from build123d import *

# Parameters (mm, degrees)
EXTRUDE_1_DEPTH     = 19.2
SKETCH_9_W          = 230
SKETCH_9_H          = 17.5
SKETCH_9_R          = 2.1
EXTRUDE_2_DEPTH     = 3
SKETCH_13_W         = 230
SKETCH_13_H         = 16
SKETCH_13_R         = 2.1
EXTRUDE_3_DEPTH     = 1.55
SKETCH_14_W         = 230
SKETCH_14_H         = 47.5
SKETCH_14_R         = 2.1
EXTRUDE_4_DEPTH     = 3
SKETCH_15_W         = 208.313471068
SKETCH_15_H         = 9.29970853
EXTRUDE_5_DEPTH     = 47.5
SKETCH_16_W         = 230
SKETCH_16_H         = 33.21324475
EXTRUDE_6_DEPTH     = 3
SKETCH_18_W         = 230
SKETCH_18_H         = 20.5
EXTRUDE_7_DEPTH     = 44.5
SKETCH_19_W         = 230
SKETCH_19_H         = 8.5
CUT_EXTRUDE_1_DEPTH = 236.542459017
CUT_EXTRUDE_2_DEPTH = 20.75


with BuildPart() as part:
    # ｽｹｯﾁ5 → ﾎﾞｽ - 押し出し1 (new body)
    with BuildSketch(Plane.XY.offset(-1.55)):
        with BuildLine():
            Line((230, -2.976), (227.539284327, -2.976))
            ThreePointArc((227.539284327, -2.976), (226.75348461, -2.728238301), (226.251905437, -2.074567596))
            Line((226.251905437, -2.074567596), (225.496824583, 0))
            Line((225.496824583, 0), (219.003175417, 0))
            Line((219.003175417, 0), (218.248094563, -2.074567596))
            ThreePointArc((218.248094563, -2.074567596), (217.74651539, -2.728238301), (216.960715673, -2.976))
            Line((216.960715673, -2.976), (214.839284327, -2.976))
            ThreePointArc((214.839284327, -2.976), (214.05348461, -2.728238301), (213.551905437, -2.074567596))
            Line((213.551905437, -2.074567596), (212.796824583, 0))
            Line((212.796824583, 0), (206.303175417, 0))
            Line((206.303175417, 0), (205.548094563, -2.074567596))
            ThreePointArc((205.548094563, -2.074567596), (205.04651539, -2.728238301), (204.260715673, -2.976))
            Line((204.260715673, -2.976), (202.139284327, -2.976))
            ThreePointArc((202.139284327, -2.976), (201.35348461, -2.728238301), (200.851905437, -2.074567596))
            Line((200.851905437, -2.074567596), (200.096824583, 0))
            Line((200.096824583, 0), (193.603175417, 0))
            Line((193.603175417, 0), (192.848094563, -2.074567596))
            ThreePointArc((192.848094563, -2.074567596), (192.34651539, -2.728238301), (191.560715673, -2.976))
            Line((191.560715673, -2.976), (189.439284327, -2.976))
            ThreePointArc((189.439284327, -2.976), (188.65348461, -2.728238301), (188.151905437, -2.074567596))
            Line((188.151905437, -2.074567596), (187.396824583, 0))
            Line((187.396824583, 0), (180.903175417, 0))
            Line((180.903175417, 0), (180.148094563, -2.074567596))
            ThreePointArc((180.148094563, -2.074567596), (179.64651539, -2.728238301), (178.860715673, -2.976))
            Line((178.860715673, -2.976), (176.739284327, -2.976))
            ThreePointArc((176.739284327, -2.976), (175.95348461, -2.728238301), (175.451905437, -2.074567596))
            Line((175.451905437, -2.074567596), (174.696824583, 0))
            Line((174.696824583, 0), (168.203175417, 0))
            Line((168.203175417, 0), (167.448094563, -2.074567596))
            ThreePointArc((167.448094563, -2.074567596), (166.94651539, -2.728238301), (166.160715673, -2.976))
            Line((166.160715673, -2.976), (164.039284327, -2.976))
            ThreePointArc((164.039284327, -2.976), (163.25348461, -2.728238301), (162.751905437, -2.074567596))
            Line((162.751905437, -2.074567596), (161.996824583, 0))
            Line((161.996824583, 0), (155.503175417, 0))
            Line((155.503175417, 0), (154.748094563, -2.074567596))
            ThreePointArc((154.748094563, -2.074567596), (154.24651539, -2.728238301), (153.460715673, -2.976))
            Line((153.460715673, -2.976), (151.339284327, -2.976))
            ThreePointArc((151.339284327, -2.976), (150.55348461, -2.728238301), (150.051905437, -2.074567596))
            Line((150.051905437, -2.074567596), (149.296824583, 0))
            Line((149.296824583, 0), (142.803175417, 0))
            Line((142.803175417, 0), (142.048094563, -2.074567596))
            ThreePointArc((142.048094563, -2.074567596), (141.54651539, -2.728238301), (140.760715673, -2.976))
            Line((140.760715673, -2.976), (138.639284327, -2.976))
            ThreePointArc((138.639284327, -2.976), (137.85348461, -2.728238301), (137.351905437, -2.074567596))
            Line((137.351905437, -2.074567596), (136.596824583, 0))
            Line((136.596824583, 0), (130.103175417, 0))
            Line((130.103175417, 0), (129.348094563, -2.074567596))
            ThreePointArc((129.348094563, -2.074567596), (128.84651539, -2.728238301), (128.060715673, -2.976))
            Line((128.060715673, -2.976), (125.939284327, -2.976))
            ThreePointArc((125.939284327, -2.976), (125.15348461, -2.728238301), (124.651905437, -2.074567596))
            Line((124.651905437, -2.074567596), (123.896824583, 0))
            Line((123.896824583, 0), (117.403175417, 0))
            Line((117.403175417, 0), (116.648094563, -2.074567596))
            ThreePointArc((116.648094563, -2.074567596), (116.14651539, -2.728238301), (115.360715673, -2.976))
            Line((115.360715673, -2.976), (113.239284327, -2.976))
            ThreePointArc((113.239284327, -2.976), (112.45348461, -2.728238301), (111.951905437, -2.074567596))
            Line((111.951905437, -2.074567596), (111.196824583, 0))
            Line((111.196824583, 0), (104.703175417, 0))
            Line((104.703175417, 0), (103.948094563, -2.074567596))
            ThreePointArc((103.948094563, -2.074567596), (103.44651539, -2.728238301), (102.660715673, -2.976))
            Line((102.660715673, -2.976), (100.539284327, -2.976))
            ThreePointArc((100.539284327, -2.976), (99.75348461, -2.728238301), (99.251905437, -2.074567596))
            Line((99.251905437, -2.074567596), (98.496824583, 0))
            Line((98.496824583, 0), (92.003175417, 0))
            Line((92.003175417, 0), (91.248094563, -2.074567596))
            ThreePointArc((91.248094563, -2.074567596), (90.74651539, -2.728238301), (89.960715673, -2.976))
            Line((89.960715673, -2.976), (87.839284327, -2.976))
            ThreePointArc((87.839284327, -2.976), (87.05348461, -2.728238301), (86.551905437, -2.074567596))
            Line((86.551905437, -2.074567596), (85.796824583, 0))
            Line((85.796824583, 0), (79.303175417, 0))
            Line((79.303175417, 0), (78.548094563, -2.074567596))
            ThreePointArc((78.548094563, -2.074567596), (78.04651539, -2.728238301), (77.260715673, -2.976))
            Line((77.260715673, -2.976), (75.139284327, -2.976))
            ThreePointArc((75.139284327, -2.976), (74.35348461, -2.728238301), (73.851905437, -2.074567596))
            Line((73.851905437, -2.074567596), (73.096824583, 0))
            Line((73.096824583, 0), (66.603175417, 0))
            Line((66.603175417, 0), (65.848094563, -2.074567596))
            ThreePointArc((65.848094563, -2.074567596), (65.34651539, -2.728238301), (64.560715673, -2.976))
            Line((64.560715673, -2.976), (62.439284327, -2.976))
            ThreePointArc((62.439284327, -2.976), (61.65348461, -2.728238301), (61.151905437, -2.074567596))
            Line((61.151905437, -2.074567596), (60.396824583, 0))
            Line((60.396824583, 0), (53.903175417, 0))
            Line((53.903175417, 0), (53.148094563, -2.074567596))
            ThreePointArc((53.148094563, -2.074567596), (52.64651539, -2.728238301), (51.860715673, -2.976))
            Line((51.860715673, -2.976), (49.739284327, -2.976))
            ThreePointArc((49.739284327, -2.976), (48.95348461, -2.728238301), (48.451905437, -2.074567596))
            Line((48.451905437, -2.074567596), (47.696824583, 0))
            Line((47.696824583, 0), (41.203175417, 0))
            Line((41.203175417, 0), (40.448094563, -2.074567596))
            ThreePointArc((40.448094563, -2.074567596), (39.94651539, -2.728238301), (39.160715673, -2.976))
            Line((39.160715673, -2.976), (37.039284327, -2.976))
            ThreePointArc((37.039284327, -2.976), (36.25348461, -2.728238301), (35.751905437, -2.074567596))
            Line((35.751905437, -2.074567596), (34.996824583, 0))
            Line((34.996824583, 0), (28.503175417, 0))
            Line((28.503175417, 0), (27.748094563, -2.074567596))
            ThreePointArc((27.748094563, -2.074567596), (27.24651539, -2.728238301), (26.460715673, -2.976))
            Line((26.460715673, -2.976), (24.339284327, -2.976))
            ThreePointArc((24.339284327, -2.976), (23.55348461, -2.728238301), (23.051905437, -2.074567596))
            Line((23.051905437, -2.074567596), (22.296824583, 0))
            Line((22.296824583, 0), (15.803175417, 0))
            Line((15.803175417, 0), (15.048094563, -2.074567596))
            ThreePointArc((15.048094563, -2.074567596), (14.54651539, -2.728238301), (13.760715673, -2.976))
            Line((13.760715673, -2.976), (11.639284327, -2.976))
            ThreePointArc((11.639284327, -2.976), (10.85348461, -2.728238301), (10.351905437, -2.074567596))
            Line((10.351905437, -2.074567596), (9.596824583, 0))
            Line((9.596824583, 0), (3.103175417, 0))
            Line((3.103175417, 0), (2.348094563, -2.074567596))
            ThreePointArc((2.348094563, -2.074567596), (1.84651539, -2.728238301), (1.060715673, -2.976))
            Line((1.060715673, -2.976), (0, -2.976))
            Line((0, -2.976), (0, -15))
            Line((0, -15), (230, -15))
            Line((230, -15), (230, -2.976))
        make_face()
    extrude(amount=-EXTRUDE_1_DEPTH)


with BuildPart() as body_2:
    # ｽｹｯﾁ9 → ﾎﾞｽ - 押し出し2 (new body)
    with BuildSketch(Plane(origin=(0, 0, -20.75), x_dir=(-1, 0, 0), z_dir=(0, 0, -1))):
        with Locations((-115, -6.25)):
            Rectangle(SKETCH_9_W, SKETCH_9_H)
        with Locations((-25, -7)):
            Circle(SKETCH_9_R, mode=Mode.SUBTRACT)
        with Locations((-85, -7)):
            Circle(SKETCH_9_R, mode=Mode.SUBTRACT)
        with Locations(Location((-145, -7, 0), (0, 0, 180))):
            Circle(SKETCH_9_R, mode=Mode.SUBTRACT)
        with Locations(Location((-205, -7, 0), (0, 0, 180))):
            Circle(SKETCH_9_R, mode=Mode.SUBTRACT)
    extrude(amount=EXTRUDE_2_DEPTH)


with BuildPart() as body_3:
    # ｽｹｯﾁ13 → ﾎﾞｽ - 押し出し3 (new, symmetric)
    with BuildSketch(Plane.XY):
        with Locations((115, -7)):
            Rectangle(SKETCH_13_W, SKETCH_13_H)
        with Locations(Location((85, -7, 0), (0, 0, 180))):
            Circle(SKETCH_13_R, mode=Mode.SUBTRACT)
        with Locations(Location((25, -7, 0), (0, 0, 180))):
            Circle(SKETCH_13_R, mode=Mode.SUBTRACT)
        with Locations((205, -7)):
            Circle(SKETCH_13_R, mode=Mode.SUBTRACT)
        with Locations((145, -7)):
            Circle(SKETCH_13_R, mode=Mode.SUBTRACT)
    extrude(amount=EXTRUDE_3_DEPTH, both=True)


with BuildPart() as body_4:
    # ﾐﾗｰ1: mirrored copy
    add(part.part.mirror(Plane.XY))


with BuildPart() as body_5:
    # Mirror 1 2: mirrored copy
    add(body_2.part.mirror(Plane.XY))


with BuildPart() as body_6:
    # ｽｹｯﾁ14 → ﾎﾞｽ - 押し出し4 (new body)
    with BuildSketch(Plane.XZ.offset(15)):
        with Locations((115, 0)):
            Rectangle(SKETCH_14_W, SKETCH_14_H)
        with Locations(Location((7, 11.15, 0), (0, 0, 180))):
            Circle(SKETCH_14_R, mode=Mode.SUBTRACT)
        with Locations((121.5, -11.15)):
            Circle(SKETCH_14_R, mode=Mode.SUBTRACT)
        with Locations((223, -11.15)):
            Circle(SKETCH_14_R, mode=Mode.SUBTRACT)
        with Locations((7, -11.15)):
            Circle(SKETCH_14_R, mode=Mode.SUBTRACT)
        with Locations(Location((223, 11.15, 0), (0, 0, 180))):
            Circle(SKETCH_14_R, mode=Mode.SUBTRACT)
        with Locations(Location((121.5, 11.15, 0), (0, 0, 180))):
            Circle(SKETCH_14_R, mode=Mode.SUBTRACT)
    extrude(amount=EXTRUDE_4_DEPTH)


with BuildPart() as body_4_1:
    add(body_4.part)

    # Combine 2: union part, body 5, body 6, body 3, body 2
    add(part.part)
    add(body_5.part)
    add(body_6.part)
    add(body_3.part)
    add(body_2.part)

    # ｽｹｯﾁ15 → ﾎﾞｽ - 押し出し5 (add)
    with BuildSketch(Plane(origin=(0, 0, -23.75), x_dir=(-1, 0, 0), z_dir=(0, 0, -1))):
        with Locations((-110.084439777, -7.625854265)):
            Rectangle(SKETCH_15_W, SKETCH_15_H)
    extrude(amount=-EXTRUDE_5_DEPTH)

    # ｽｹｯﾁ16 → ﾎﾞｽ - 押し出し6 (add)
    with BuildSketch(Plane.XZ.offset(18)):
        with Locations((115, 1.195676811)):
            Rectangle(SKETCH_16_W, SKETCH_16_H)
    extrude(amount=-EXTRUDE_6_DEPTH)

    # ｽｹｯﾁ18 → ﾎﾞｽ - 押し出し7 (add)
    with BuildSketch(Plane.XY.offset(23.75)):
        with Locations((115, -7.75)):
            Rectangle(SKETCH_18_W, SKETCH_18_H)
    extrude(amount=-EXTRUDE_7_DEPTH)

    # ｽｹｯﾁ19 → ｶｯﾄ - 押し出し1 (cut, through all)
    with BuildSketch(Plane.XY.offset(23.75)):
        with Locations((115, -1.75)):
            Rectangle(SKETCH_19_W, SKETCH_19_H)
    extrude(amount=-CUT_EXTRUDE_1_DEPTH, mode=Mode.SUBTRACT)

    # ｽｹｯﾁ17 → ｶｯﾄ - 押し出し2 (cut, symmetric)
    with BuildSketch(Plane.XY):
        Polygon((5.88, 0), (26.88, 0), (21.38, -10), (11.38, -10), align=None)
        Polygon((55.19, 0), (76.19, 0), (70.69, -10), (60.69, -10), align=None)
        Polygon((104.5, 0), (125.5, 0), (120, -10), (110, -10), align=None)
        Polygon((153.81, 0), (174.81, 0), (169.31, -10), (159.31, -10), align=None)
        Polygon((203.12, 0), (224.12, 0), (218.62, -10), (208.62, -10), align=None)
    extrude(amount=CUT_EXTRUDE_2_DEPTH, both=True, mode=Mode.SUBTRACT)


solid = body_4_1.part
Can you work these out from the model? Positions are in its coordinate system, mm. A direction names the side the tool comes from. Give positions to 0.01 mm unless a question says otherwise; leave off trailing zeros. Loops run counter-clockwise (first coordinate to the right, second up) from the corner with the lowest first, then second, coordinate; pieces in that order, holes last. Notation, with made-up numbers: M -6,64 L 39,64 A11 cw 39,83 Z; hole C 71,-38.75 d6. An arc over 180 degrees is marked long. One line per item, written item: value. Start each with the question number.
1) If I drill on line 1 (X direction, y = -6.5, z = -0.5) (3 decimals); line 2 (X direction, y = -7.25, z = -9); line 3 (Z direction, x = 18.5, y = -7), over which ranges is the centre line in solid material (lowest first)? Write a range as [from, to].
2) If we section it at C-C, the plane x = 63: Write out the boundary of the cut face in (y, z).
3) If we section it at A-A, the plane y = -8: Write out the boundary of the cut face in (x, z), and give its area (3 significant figures).
4) I'm going to push a flat-ended pin straight in: pin 1 (3 mm diameter, centred on x = 114.5, z = 4.5, fed in from +Y). Where does the tip first touch, or does it pass through?
5) If we section it at B-B, the plane z = -16.5: Write out the boundary of the cut face in (x, y).
6) Thinking about a two-plate mould opening in X: for faces 3 (the face through (113, -6, -21)), 4 (the face through (0, -12, 0)), 5 (the face through (219.735, -7.972, 0.291)), 6 (the face through (66, -10, 0)), which applies, +X half, -X half, draft (parallel to the pull), parting line (faces both ways), or undercut?
7) On a 3-axis mill with a long thin cutter (end or side, diameter ignored), from which of +Z, -Z, +X, -X, +Y, -Y can I reach the whole of each face in a straight line? I mean faces 1 (the face through (113, -18, 0)), 2 (the face through (10.295, -8.028, -0.291)). Say none if no direction works.
Completed:
1. line 1: x = [0, 9.455], [23.305, 58.765], [72.615, 108.075], [121.925, 157.385], [171.235, 206.695], [220.545, 230]
1. line 2: x = [0, 9.87], [22.89, 59.18], [72.2, 108.49], [121.51, 157.8], [170.82, 207.11], [220.13, 230]
1. line 3: z = [-23.75, -20.75], [20.75, 23.75]
2. outline: M -18,-23.75 L -6,-23.75 L -6,-20.75 L -10,-20.75 L -10,20.75 L -6,20.75 L -6,23.75 L -18,23.75 Z
3. outline: M 0,-23.75 L 230,-23.75 L 230,23.75 L 0,23.75 Z; hole M 10.28,-20.75 L 22.48,-20.75 L 22.48,20.75 L 10.28,20.75 Z; hole M 59.59,-20.75 L 71.79,-20.75 L 71.79,20.75 L 59.59,20.75 Z; hole M 108.9,-20.75 L 121.1,-20.75 L 121.1,20.75 L 108.9,20.75 Z; hole M 158.21,-20.75 L 170.41,-20.75 L 170.41,20.75 L 158.21,20.75 Z; hole M 207.52,-20.75 L 219.72,-20.75 L 219.72,20.75 L 207.52,20.75 Z
3. area: 8,390 mm^2
4. pin 1: stops at y = -10
5. outline: M 0,-18 L 230,-18 L 230,-6 L 220.82,-6 L 218.62,-10 L 208.62,-10 L 206.42,-6 L 171.51,-6 L 169.31,-10 L 159.31,-10 L 157.11,-6 L 122.2,-6 L 120,-10 L 110,-10 L 107.8,-6 L 72.89,-6 L 70.69,-10 L 60.69,-10 L 58.49,-6 L 23.58,-6 L 21.38,-10 L 11.38,-10 L 9.18,-6 L 0,-6 Z
6. face 3: draft
6. face 4: -X half
6. face 5: undercut
6. face 6: undercut
7. face 1: +Z, -Z, +X, -X, -Y
7. face 2: +Y
